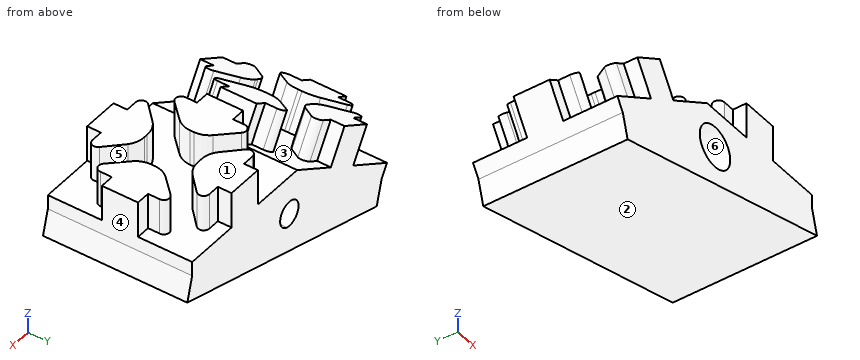
from build123d import *

# Parameters (mm, degrees)
SKIZZE1_W                       = 20
SKIZZE1_H                       = 20
AUFSATZ_LINEAR_AUSTRAGEN1_DEPTH = 2
AUFSATZ_LINEAR_AUSTRAGEN3_DEPTH = 5
VERRUNDUNG1_R                   = 3
VERRUNDUNG1_OF_SPIEGELN1_R      = 3
AUFSATZ_LINEAR_AUSTRAGEN4_REACH = 35.564
SKIZZE3_W                       = 37.447689889
SKIZZE3_H                       = 20
SCHNITT_LINEAR_AUSTRAGEN1_DEPTH = 32.884097459
SKIZZE4_3_R                     = 2.9
SKIZZE4_3_R_2                   = 1.75
SCHNITT_LINEAR_AUSTRAGEN2_DEPTH = 16


with BuildPart() as part:
    # Skizze1 → Aufsatz-Linear austragen1 (new body)
    with BuildSketch(Plane.XY):
        with Locations((10, 10)):
            Rectangle(SKIZZE1_W, SKIZZE1_H)
    aufsatz_linear_austragen1 = extrude(amount=AUFSATZ_LINEAR_AUSTRAGEN1_DEPTH)

    # Skizze2 → Aufsatz-Linear austragen3 (add)
    with BuildSketch(Plane.XY.offset(2)):
        with BuildLine():
            Line((12.5, 18.1), (12.5, 20))
            Line((12.5, 20), (7.5, 20))
            Line((7.5, 20), (7.5, 18.1))
            Line((7.5, 18.1), (5.883086579, 18.1))
            ThreePointArc((5.883086579, 18.1), (5.159199271, 17.610494692), (5.343893194, 16.756377348))
            Line((5.343893194, 16.756377348), (8.350270542, 13.75))
            Line((8.350270542, 13.75), (11.649729458, 13.75))
            Line((11.649729458, 13.75), (14.656106806, 16.756377348))
            ThreePointArc((14.656106806, 16.756377348), (14.840800729, 17.610494692), (14.116913421, 18.1))
            Line((14.116913421, 18.1), (12.5, 18.1))
        make_face()
        with BuildLine():
            Line((1.9, 12.5), (0, 12.5))
            Line((0, 12.5), (0, 7.5))
            Line((0, 7.5), (1.9, 7.5))
            Line((1.9, 7.5), (1.9, 5.883086579))
            ThreePointArc((1.9, 5.883086579), (2.389505308, 5.159199271), (3.243622652, 5.343893194))
            Line((3.243622652, 5.343893194), (5.46777943, 7.668819976))
            ThreePointArc((5.46777943, 7.668819976), (6.084181953, 8.625353412), (6.3, 9.742640687))
            Line((6.3, 9.742640687), (6.3, 10.257359313))
            ThreePointArc((6.3, 10.257359313), (6.084181953, 11.374646588), (5.46777943, 12.331180024))
            Line((5.46777943, 12.331180024), (3.243622652, 14.656106806))
            ThreePointArc((3.243622652, 14.656106806), (2.389505308, 14.840800729), (1.9, 14.116913421))
            Line((1.9, 14.116913421), (1.9, 12.5))
        make_face()
        with BuildLine():
            Line((7.5, 0), (12.5, 0))
            Line((12.5, 0), (12.5, 1.9))
            Line((12.5, 1.9), (14.116913421, 1.9))
            ThreePointArc((14.116913421, 1.9), (14.840800729, 2.389505308), (14.656106806, 3.243622652))
            Line((14.656106806, 3.243622652), (12.366329752, 5.533399706))
            ThreePointArc((12.366329752, 5.533399706), (11.386219612, 6.121310843), (10.257359313, 6.3))
            Line((10.257359313, 6.3), (9.742640687, 6.3))
            ThreePointArc((9.742640687, 6.3), (8.613780388, 6.121310843), (7.633670248, 5.533399706))
            Line((7.633670248, 5.533399706), (5.343893194, 3.243622652))
            ThreePointArc((5.343893194, 3.243622652), (5.159199271, 2.389505308), (5.883086579, 1.9))
            Line((5.883086579, 1.9), (7.5, 1.9))
            Line((7.5, 1.9), (7.5, 0))
        make_face()
        with BuildLine():
            Line((20, 7.5), (20, 12.5))
            Line((20, 12.5), (18.1, 12.5))
            Line((18.1, 12.5), (18.1, 14.116913421))
            ThreePointArc((18.1, 14.116913421), (17.610494692, 14.840800729), (16.756377348, 14.656106806))
            Line((16.756377348, 14.656106806), (14.53222057, 12.331180024))
            ThreePointArc((14.53222057, 12.331180024), (13.915818047, 11.374646588), (13.7, 10.257359313))
            Line((13.7, 10.257359313), (13.7, 9.742640687))
            ThreePointArc((13.7, 9.742640687), (13.915818047, 8.625353412), (14.53222057, 7.668819976))
            Line((14.53222057, 7.668819976), (16.756377348, 5.343893194))
            ThreePointArc((16.756377348, 5.343893194), (17.610494692, 5.159199271), (18.1, 5.883086579))
            Line((18.1, 5.883086579), (18.1, 7.5))
            Line((18.1, 7.5), (20, 7.5))
        make_face()
    aufsatz_linear_austragen3 = extrude(amount=AUFSATZ_LINEAR_AUSTRAGEN3_DEPTH)

    # Verrundung1
    verrundung1_edges = [part.edges().sort_by_distance(p)[0] for p in [
        (8.350270542, 13.75, 4.5),
        (11.649729458, 13.75, 4.5),
    ]]
    fillet(verrundung1_edges, radius=VERRUNDUNG1_R)

    # Spiegeln1: Aufsatz-Linear austragen1, Aufsatz-Linear austragen3 across plane
    add(aufsatz_linear_austragen1.mirror(Plane(origin=(0.518393786, 0, 0.144857975), x_dir=(-0.2691263412444344, 0, 0.963104881333484), z_dir=(-0.9631048813334839, 0, -0.2691263412444344))))
    add(aufsatz_linear_austragen3.mirror(Plane(origin=(0.518393786, 0, 0.144857975), x_dir=(-0.2691263412444344, 0, 0.963104881333484), z_dir=(-0.9631048813334839, 0, -0.2691263412444344))))

    # Verrundung1 of Spiegeln1
    verrundung1_of_spiegeln1_edges = [part.edges().sort_by_distance(p)[0] for p in [
        (-8.436651724, 13.75, -0.190873297),
        (-11.258157703, 13.75, -1.901292296),
    ]]
    fillet(verrundung1_of_spiegeln1_edges, radius=VERRUNDUNG1_OF_SPIEGELN1_R)

    # Skizze3 → Aufsatz-Linear austragen4 (add, up to next)
    with BuildSketch(Plane(origin=(2.36988033, 0, -8.480936141), x_dir=(-0.963104881333484, 0, -0.26912634124443463), z_dir=(0.26912634124443463, 0, -0.963104881333484)), mode=Mode.PRIVATE) as aufsatz_linear_austragen4_sk1:
        with Locations((-0.538252683, 10)):
            Rectangle(SKIZZE3_W, SKIZZE3_H)
    aufsatz_linear_austragen4_tool1 = extrude(aufsatz_linear_austragen4_sk1.sketch, amount=-AUFSATZ_LINEAR_AUSTRAGEN4_REACH, mode=Mode.PRIVATE) - part.part
    add(aufsatz_linear_austragen4_tool1.solids().sort_by_distance((2.888274, 10, -8.336078))[0])

    # Skizze4 → Schnitt-Linear austragen1 (cut, through all)
    with BuildSketch(Plane.XZ):
        with BuildLine():
            ThreePointArc((3.245339923, -3.351275437), (2.553238921, -1.957234652), (1.024368826, -1.665841895))
            Line((1.024368826, -1.665841895), (1.966311021, -5.03670898))
            ThreePointArc((1.966311021, -5.03670898), (2.889380708, -4.409174435), (3.245339923, -3.351275437))
        make_face()
        with BuildLine():
            Line((1.966311021, -5.03670898), (1.024368826, -1.665841895))
            ThreePointArc((1.024368826, -1.665841895), (-0.190093619, -3.822246535), (1.966311021, -5.03670898))
        make_face()
    extrude(amount=-SCHNITT_LINEAR_AUSTRAGEN1_DEPTH, mode=Mode.SUBTRACT)

    # Skizze4<3> → Schnitt-Linear austragen2 (cut)
    with BuildSketch(Plane.XZ):
        with Locations(Location((1.495339923, -3.351275437, 0), (0, 0, 270))):
            Circle(SKIZZE4_3_R)
        with Locations(Location((1.495339923, -3.351275437, 0), (0, 0, 270))):
            Circle(SKIZZE4_3_R_2, mode=Mode.SUBTRACT)
    extrude(amount=-SCHNITT_LINEAR_AUSTRAGEN2_DEPTH, mode=Mode.SUBTRACT)


solid = part.part
Geometry: final body of the model. Coordinates: model frame, mm. Face numbers are marked on the shaded views. A direction names the side the tool comes from. Coordinates: 2 decimals unless noted, no trailing zeros. Loops run counter-clockwise (first coordinate to the right, second up) from the corner with the lowest first, then second, coordinate; pieces in that order, holes last. Notation, with made-up numbers: M -2.75,4 L 49.25,4 A16 cw 49.25,35 Z; hole C 63,31 d11. An arc over 180 degrees is marked long. One line per item, written item: value. Start each with the question number.
1) Reachability of the marked faces 4, 5 and 6 from +Z, -Z, +X, -X, +Y, -Y: full face, straight path, thin tool, end or side. Return the list, or none.
2) Cut plane C-C (y = 4.5). Return loops of the section in (x, z), then the cut area to 3 significant figures.
3) Cut plane B-B (x = 13). Return loops of the section in (y, z).
4) Draft query along Z for the marked faces 1, 2 and 3. Return one class per face: released by +Z, released by -Z, zero draft, split by the parting line, or undercut.
5) Material intervals for L1, parallel to X at y = 12.5, z = -2; L2, parallel to X at y = 7.25, z = -3.25; L3, parallel to X at y = 18.75, z = -2.5, sorted ascending. Write a range as from..to.
6) Pin query (flat end, axial travel): P1, Ø2, axis at y = 16, z = 2, coming from the -X side; P2, Ø2, axis at x = 19.5, z = 3.5, coming from the +Y side; P3, Ø1.5, axis at x = 0.5, z = 5.5, coming from the -Y side. Return the tip coordinate at first contact, or that it passes through.
7) Cut plane A-A (y = 2.5). Return loops of the section in (x, z).
8) Cut plane D-D (z = -11). Return loops of the section in (x, y), then the cut area to 3 significant figures.
Evaluation:
1. face 4: +Z, +X, +Y, -Y
1. face 5: +Z
1. face 6: -Y
2. outline: M -17.1,-8.37 L -16.07,-10.08 L -15.14,-13.38 L 20.92,-3.3 L 20,0 L 20,2 L 13.4,2 L 13.4,7 L 6.6,7 L 6.6,2 L 0,2 L -5.64,-1.42 L -8.24,2.85 L -14.05,-0.67 L -11.46,-4.95 Z; hole C 1.5,-3.35 d5.8
2. area: 347 mm^2
3. outline: M 0,-5.51 L 20,-5.51 L 20,2 L 18.1,2 L 18.1,7 L 15.1,7 L 15.1,2 L 4.9,2 L 4.9,7 L 1.9,7 L 1.9,2 L 0,2 Z
4. face 1: released by +Z
4. face 2: released by -Z
4. face 3: undercut
5. L1: -16.24..-14.76, -6.6..-1.07, 4.06..20.56
5. L2: -17.98..-14.28, -8.66..-1.4, 4.39..20.91
5. L3: -11.89..-0.03, 3.02..20.7
6. P1: x = -11.29
6. P2: y = 12.5
6. P3: y = 7.5
7. outline: M -17.1,-8.37 L -16.07,-10.08 L -15.14,-13.38 L 20.92,-3.3 L 20,0 L 20,2 L 14.88,2 L 14.88,7 L 5.12,7 L 5.12,2 L 0,2 L -4.38,-0.66 L -6.97,3.62 L -15.31,-1.44 L -12.72,-5.71 Z; hole C 1.5,-3.35 d5.8
8. outline: M -15.81,0 L -6.64,0 L -6.64,20 L -15.81,20 Z
8. area: 183 mm^2
